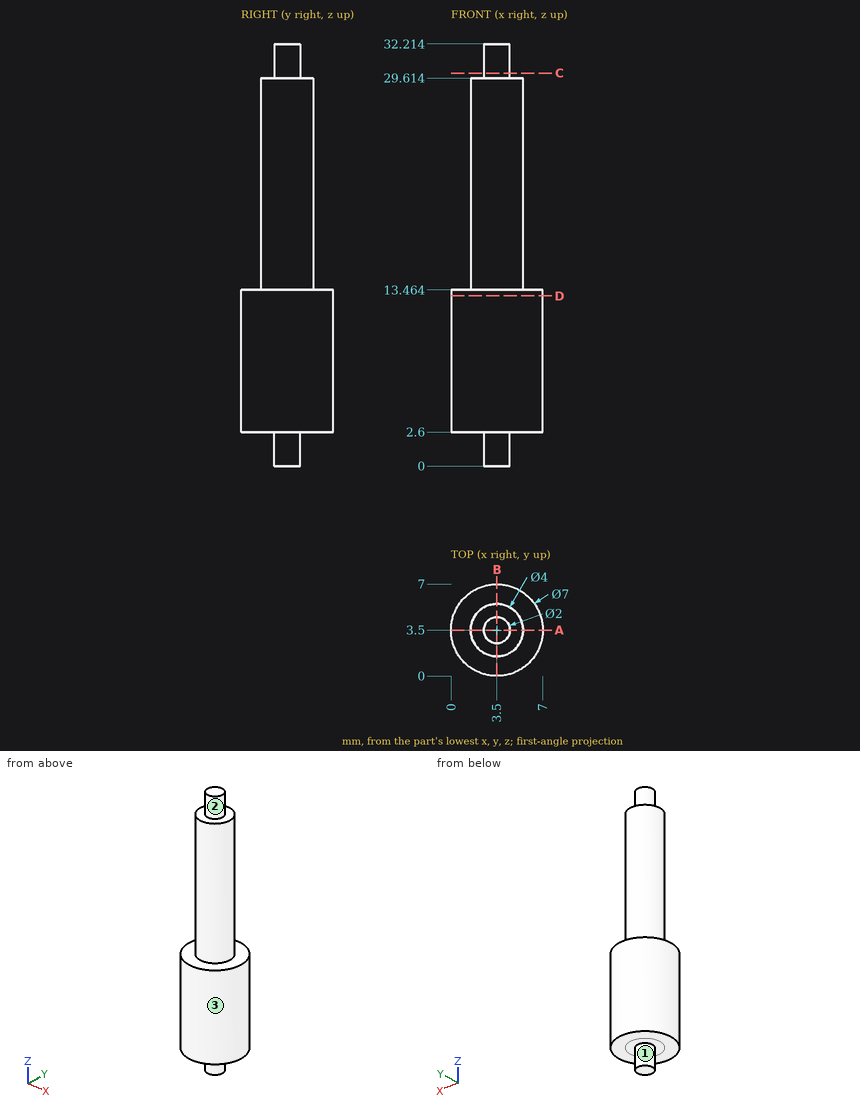
Geometry check sheet. Reference: drawing and pictorial views, mm from the part's lowest x, y, z. A direction names the side the tool comes from. Give positions to 0.01 mm unless a question says otherwise; leave off trailing zeros. Order: outer loops, then holes, each group sorted by start corner. A loop starts at its lowest first (then second) coordinate and runs counter-clockwise, first axis right, second up.
1. Gauge pin test, flat end, axial feed: pin 1 Ø3 at (x, z) = (0.5, 27) entering from -Y. Record the tip position at first contact, or that the pin passes through.
2. Section check A-A, the plane y = 3.5. Enter the section's corners in (x, z), and give its area (3 significant figures).
3. Section check D-D, the plane z = 13. Enter the section's corners in (x, y), and give its area (3 significant figures).
4. Access from +Z, -Z, +X, -X, +Y, -Y to the whole of each face (thin tool, end or side, straight path). Record for the marked faces 1, 2 and 3.
5. Section check C-C, the plane z = 30. Enter the section's corners in (x, y).
6. Thickness scan on L1, parallel to Z at x = 6.5, y = 2.25; L2, parallel to Z at x = 2, y = 4; L3, parallel to Y at x = 2.25, z = 24.5. Record the ranges inside material, lowest first.
Values follow:
1. pin 1: stops at y = 2.18
2. outline: (0, 2.6) - (2.5, 2.6) - (2.5, 0) - (4.5, 0) - (4.5, 2.6) - (7, 2.6) - (7, 13.46) - (5.5, 13.46) - (5.5, 29.61) - (4.5, 29.61) - (4.5, 32.21) - (2.5, 32.21) - (2.5, 29.61) - (1.5, 29.61) - (1.5, 13.46) - (0, 13.46) - close
2. area: 151 mm2
3. outline: circle Ø7 at (3.5, 3.5)
3. area: 38.5 mm2
4. face 1: -Z
4. face 2: +Z
4. face 3: +Z, -Z
5. outline: circle Ø2 at (3.5, 3.5)
6. L1: z = 2.6 to 13.46
6. L2: z = 2.6 to 29.61
6. L3: y = 1.94 to 5.06
